Can you work these out from the model? Positions are in its coordinate system, mm. Face numbers are marked on the shaded views. Coordinates: 2 decimals unless noted, no trailing zeros. Order: outer loops, then holes, each group sorted by start corner. A loop starts at its lowest first (then second) coordinate and runs counter-clockwise, first axis right, second up. Notation, with made-up numbers: (54, -13.5) - (111, -13.5) arc R30 cw to (111, 23.5) - close; hole circle Ø10 at (-19, 47.5). An arc over 180 degrees is marked (long way). Use a Markdown table: item, result. Add a question column.
(1) I want a section at B-B (z = 54). List the corners of the cut face in (x, y) for me.
(2) We'd pull the mould along X, two halves only. Please class the marked faces 1, 2 and 3: pulls with the +X half, pulls with the -X half, needs draft (parallel to the pull), parting line crosses it, or undercut.
(3) If I drill on L1, parallel to Z at x = 14.5, y = -44.5; L2, parallel to Y at x = 0, z = 11; L3, parallel to X at y = 0, z = 9, over which ranges is the centre line in solid material (lowest first)? Write a range as [from, to].
(4) For pin 1 Ø6 at (y, z) = (10, 20.5) entering from -X; pin 2 Ø1.5 at (x, y) = (-62, -36) entering from +Z; pin 3 Ø3 at (y, z) = (46, 26) entering from +X, each with a flat end and sliding along its axis, tell me the tip position at first contact or that it passes through.
(5) I want a section at A-A (z = 21.5). List the corners of the cut face in (x, y) for me.
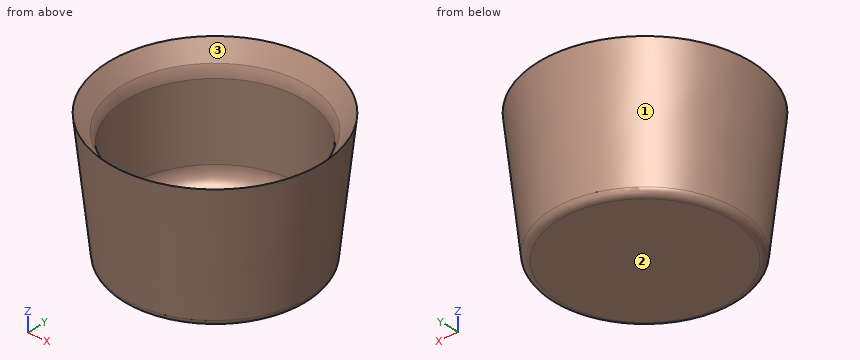
```python
from build123d import *

# Parameters (mm, degrees)
F2_R = 12.7
F3_R = 5.08


with BuildPart() as f1:
    # F0 (on Right) → F1 (revolve)
    with BuildSketch(Plane.YZ):
        Polygon((-65.786, 44.882439), (-78.269736, 60.014239), (-67.727208, -36.489587), (0, -36.489587), (0, -28.506783), (-65.786, -28.506783), align=None)
    revolve(axis=Axis((0, 0, -32.498185), (0, 0, -1)))

    # F2
    f2_edges = [f1.edges().sort_by_distance(p)[0] for p in [
        (0, 65.786, -28.506783),
        (0, 65.786, 44.882439),
        (0, -65.786, 8.187828),
    ]]
    fillet(f2_edges, radius=F2_R)

    # F3
    f3_edges = [f1.edges().sort_by_distance(p)[0] for p in [
        (0, 67.727208, -36.489587),
    ]]
    fillet(f3_edges, radius=F3_R)


solid = f1.part
```
Answers follow:
| question | item | result |
|---|---|---|
| 1 | outline | circle Ø155.23 at (0, 0); hole circle Ø146.62 at (0, 0) |
| 2 | face 1 | parting line crosses it |
| 2 | face 2 | needs draft |
| 2 | face 3 | undercut |
| 3 | L1 | z = [-36.49, -28.51] |
| 3 | L2 | y = [-72.92, -65.79], [65.79, 72.92] |
| 3 | L3 | x = [-72.7, -65.79], [65.79, 72.7] |
| 4 | pin 1 | stops at x = -73.77 |
| 4 | pin 2 | stops at z = 52.95 |
| 4 | pin 3 | stops at x = 59.84 |
| 5 | outline | circle Ø148.12 at (0, 0); hole circle Ø131.57 at (0, 0) |
